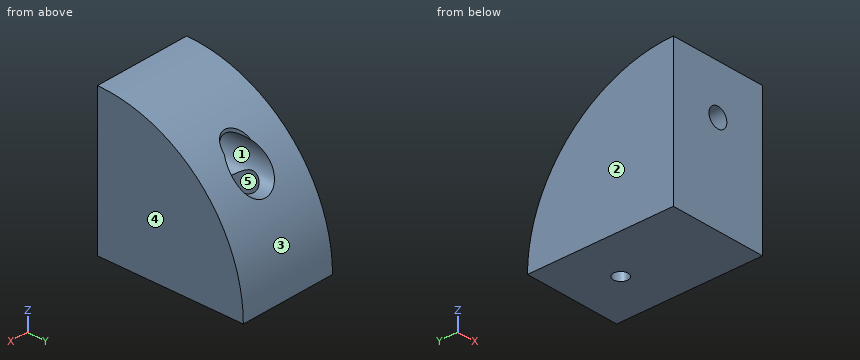
Autodesk Inventor part; units mm, degrees
ref_plane "工作平面1" through (0, 30, 0) normal (0, -1, 0) x (1, 0, 0)
ref_plane "工作平面2" through (10, 0, 30) normal (0, 0, -1) x (-1, 0, 0)
ref_plane "YZ Plane" through (0, 0, 0) normal (1, 0, 0) x (0, 1, 0)
sketch "草圖1" plane through (0, 0, 0) normal (1, 0, 0) x (0, 1, 0)
  line L0 (0, 0) -> (0, 30)
  arc A0 (30, 0) -> (0, 30) centre (0, 0) ccw
  line L1 (30, 0) -> (0, 0)
  dimension "d0" = 30
extrude "擠出1" add sketch "草圖1" along normal blind 20
ref_plane "工作平面1" through (0, 30, 0) normal (0, -1, 0) x (1, 0, 0)
sketch "草圖2" plane through (0, 30, 0) normal (0, -1, 0) x (1, 0, 0)
  line L0 (0, 0) -> (20, 0)
  point P0 (10, 20)
  point P1 (10, 0)
  dimension "d3" = 20
hole "孔1" at (10, 30, 20) direction (0, -1, 0) diameter 4 end through all counterbore diameter 8 counterbore depth 25
ref_plane "工作平面2" through (10, 0, 30) normal (0, 0, -1) x (-1, 0, 0)
sketch "草圖3" plane through (10, 0, 30) normal (0, 0, -1) x (-1, 0, 0)
  line L0 (10, 0) -> (-10, 0)
  point P0 (0, 20)
  point P1 (0, 0)
  dimension "d11" = 20
hole "孔2" at (10, 20, 30) direction (0, 0, -1) diameter 3 end through all counterbore diameter 6 counterbore depth 25
properties part number "鋁擠固定器小"
Check sheet for the modelled part. Datum: model origin and axes. Units: mm. Face numbers are marked on the shaded views. A direction names the side the tool comes from. Give positions to 0.01 mm unless a question says otherwise; leave off trailing zeros. Write each loop counter-clockwise with the first axis right and the second up, starting at its lowest first coordinate (ties: lowest second). Pieces come first, ordered by that corner, then holes. Notation, with made-up numbers: (45, -10) -> (74, -10) arc R30 cw to (74, 20) -> close; hole circle Ø7 at (87.5, 71.5). An arc over 180 degrees is marked (long way). Use CSV: the item, a comma, the result in double quotes. Start each with the question number.
Q1. Cross-section at A-A on x = 10. Enter the section's corners in (y, z).
Q2. Depth check by flat-ended pin: P1, Ø2, axis at x = 17, z = 6, coming from the +Y side; P2, Ø3.5, axis at x = 10, z = 20, coming from the -Y side; P3, Ø5, axis at x = 10, y = 19, coming from the +Z side; P4, Ø1, axis at x = 4.5, z = 25, coming from the +Y side. Enter the tip coordinate at first touch or a pass-through.
Q3. Scan lines: line 1 along X through (y, z) = (3.1, 20); line 2 along X through (y, z) = (20, 9); line 3 along Z through (x, y) = (10, 10.5). Record each from-to range of solid material in increasing order.
Q4. Release check for a two-part mould opening along Z. For the marked faces 1, 2 and 3 record: +Z half, -Z half, draft (parallel to the pull), parting line (faces both ways), or undercut.
Q5. Cross-section at D-D on z = 12. Enter the section's corners in (x, y).
Q6. Cross-section at B-B on z = 21. Enter the section's corners in (x, y), and give its area (3 significant figures).
Q7. Tool access check on the marked faces 4 and 5. Record the directions out of +Z, -Z, +X, -X, +Y, -Y that give a thin tool (end or side, any length) a straight path to the whole face; none if there is none.
Q8. Cross-section at C-C on y = 19. Enter the section's corners in (x, z), and give its area (3 significant figures).
Working result:
1,outline,"(0, 0) -> (18.5, 0) -> (18.5, 5) -> (17, 5) -> (17, 16) -> (5, 16) -> (5, 18) -> (0, 18) -> close; (0, 22) -> (5, 22) -> (5, 24) -> (17, 24) -> (17, 24.72) arc R30 ccw to (0, 30) -> close; (21.5, 0) -> (30, 0) arc R30 ccw to (25.38, 16) -> (23, 16) -> (23, 5) -> (21.5, 5) -> close"
2,P1,"stops at y = 29.58"
2,P2,"passes through"
2,P3,"stops at z = 25.05"
2,P4,"stops at y = 17.31"
3,line 1,"x = 0 to 8, 12 to 20"
3,line 2,"x = 0 to 7, 13 to 20"
3,line 3,"z = 0 to 16, 24 to 28.1"
4,face 1,"undercut"
4,face 2,"draft"
4,face 3,"+Z half"
5,outline,"(0, 0) -> (20, 0) -> (20, 27.5) -> (0, 27.5) -> close; hole circle Ø6 at (10, 20)"
6,outline,"(0, 0) -> (8.27, 0) -> (8.27, 5) -> (6.13, 5) -> (6.13, 21.42) -> (0, 21.42) -> close; (11.73, 0) -> (20, 0) -> (20, 21.42) -> (13.87, 21.42) -> (13.87, 5) -> (11.73, 5) -> close"
6,area,"284 mm^2"
7,face 4,"+Z, -Z, +X, +Y, -Y"
7,face 5,"+Z"
8,outline,"(0, 0) -> (8.88, 0) -> (8.88, 5) -> (7.17, 5) -> (7.17, 17.17) arc R4 cw to (7.17, 22.83) -> (7.17, 23.22) -> (0, 23.22) -> close; (11.12, 0) -> (20, 0) -> (20, 23.22) -> (12.83, 23.22) -> (12.83, 22.83) arc R4 cw to (12.83, 17.17) -> (12.83, 5) -> (11.12, 5) -> close"
8,area,"341 mm^2"
